Geometry: final body of the model. Coordinates: model frame, mm. A direction names the side the tool comes from. Give positions to 0.01 mm unless a question says otherwise; leave off trailing zeros. Write each loop counter-clockwise with the first axis right and the second up, starting at its lowest first coordinate (ties: lowest second). Pieces come first, ordered by that corner, then holes. Notation, with made-up numbers: (26, -33) -> (50, -33) arc R29 ccw to (50, -11) -> close; hole circle Ø5 at (8.25, 65). An arc over 180 degrees is marked (long way). Answer as a JSON object with one key per item and string values.
from build123d import *

# Parameters (mm, degrees)
SKETCH1_R           = 2.5
BOSS_EXTRUDE1_DEPTH = 9.525
SKETCH2_R           = 3
BOSS_EXTRUDE2_DEPTH = 1
FILLET1_R           = 1.8


with BuildPart() as part:
    # Sketch1 → Boss-Extrude1 (new body)
    with BuildSketch(Plane(origin=(0, 0, 0), x_dir=(1, 0, 0), z_dir=(0, 1, 0))):
        Circle(SKETCH1_R)
    extrude(amount=BOSS_EXTRUDE1_DEPTH)

    # Sketch2 → Boss-Extrude2 (add)
    with BuildSketch(Plane.XZ):
        Circle(SKETCH2_R)
    extrude(amount=BOSS_EXTRUDE2_DEPTH)

    # Fillet1
    fillet1_edges = [part.edges().sort_by_distance(p)[0] for p in [
        (-2.5, 9.525, 0),
    ]]
    fillet(fillet1_edges, radius=FILLET1_R)


solid = part.part
Q1. Cut plane A-A (y = 3.5). Return the cut outline in (x, z), and give its area (3 significant figures).
Values:
{"outline": "circle Ø5 at (0, 0)", "area": "19.6 mm²"}
Q2. Set-up query: faces 1 (the flat face through (0, -1, 0)), 2 (the flat face through (-2, 0, 2)). Return all of +Z, -Z, +X, -X, +Y, -Y with unobstructed straight access to the full face (end or side cutting, diameter ignored); none if empty.
Values:
{"face 1": "+Z, -Z, +X, -X, -Y", "face 2": "+Y"}
Q3. First-contact query: P1, Ø1, axis at y = 2, z = 0.5, coming from the +X side; P2, Ø3, axis at x = -1, y = 4, coming from the -Z side. Flat tips, straight axial feed; report the tip coordinate or a pass-through.
Values:
{"P1": "x = 2.5", "P2": "z = -2.5"}
Q4. Material intervals for L1, parallel to Y at x = -2.2, z = -1.75; L2, parallel to X at y = 6, z = 0, sorted ascending. Write a range as from..to.
Values:
{"L1": "-1..0", "L2": "-2.5..2.5"}
